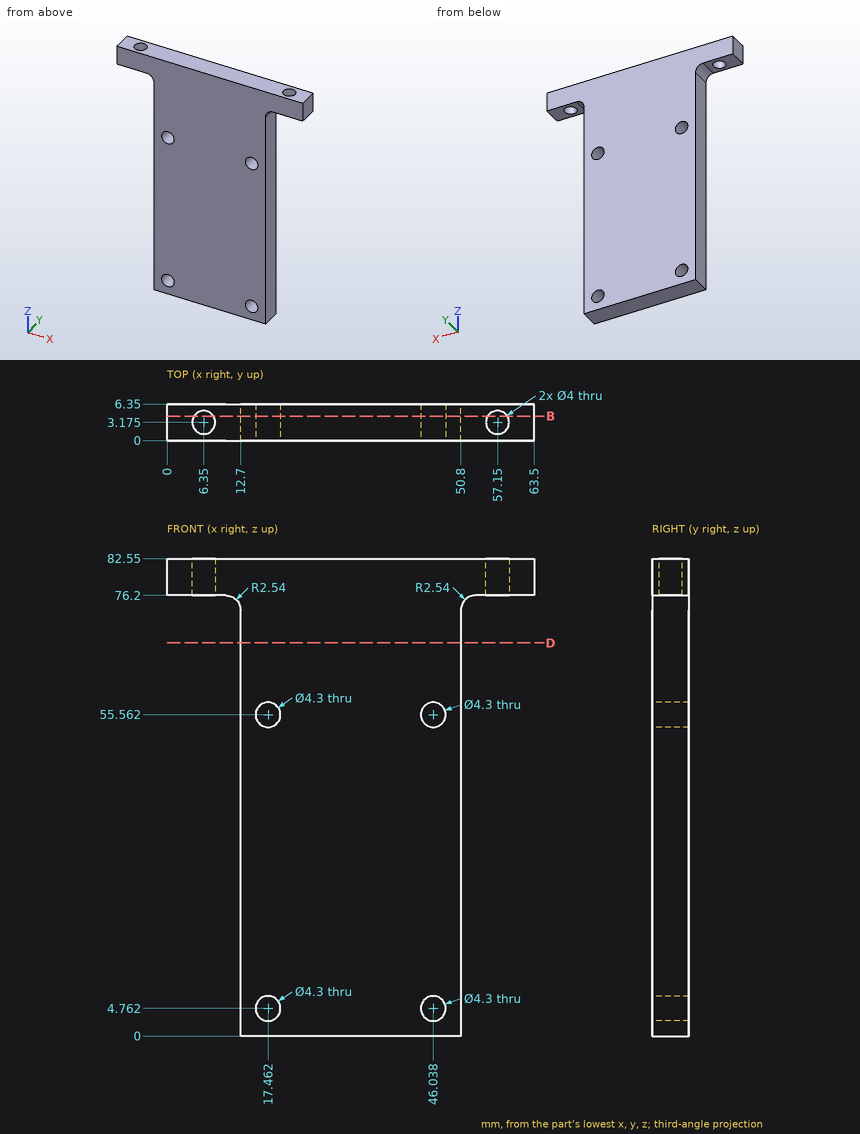
Geometry: see drawing. Coordinates: mm, zero at the bounding-box minimum. Round coordinates to 2 decimals unless told otherwise and drop trailing zeros. Write each loop counter-clockwise with the first axis right and the second up, starting at its lowest first coordinate (ties: lowest second). Pieces come first, ordered by that corner, then holes. Notation, with made-up numbers: (-1, 22.25) - (52, 22.25) arc R18 cw to (52, 48.25) - close; hole circle Ø9 at (29.25, 9). An arc over 180 degrees is marked (long way). Use CSV: the item, a comma, the result in double quotes. Start each with the question number.
(1) First-contact query: pin 1 Ø3.5 at (x, z) = (17.46, 55.56) entering from -Y; pin 2 Ø3 at (x, y) = (3.5, 2) entering from -Z; pin 3 Ø1.9 at (y, z) = (2, 48.5) entering from +X. Flat tips, straight axial feed; report the tip coordinate or a pass-through.
(2) Material intervals for probe 1 along Z at (x, y) = (46, 5.5); probe 2 along X at (y, z) = (2, 57) (1 decimal); probe 3 along X at (y, z) = (3.75, 16), sorted ascending. Write a range as [from, to].
(3) Cut plane B-B, the plane y = 4.25. Return loops of the section in (x, z), and give its area (3 significant figures).
(4) Cut plane D-D, the plane z = 68. Return loops of the section in (x, y), and give its area (3 significant figures).
Geometry says:
1,pin 1,"through"
1,pin 2,"z = 76.2"
1,pin 3,"x = 50.8"
2,probe 1,"[0, 2.61], [6.91, 53.41], [57.71, 82.55]"
2,probe 2,"[12.7, 15.9], [19.1, 44.4], [47.6, 50.8]"
2,probe 3,"[12.7, 50.8]"
3,outline,"(0, 76.2) - (4.66, 76.2) - (4.66, 82.55) - (0, 82.55) - close; (8.04, 76.2) - (10.16, 76.2) arc R2.54 cw to (12.7, 73.66) - (12.7, 0) - (50.8, 0) - (50.8, 73.66) arc R2.54 cw to (53.34, 76.2) - (55.46, 76.2) - (55.46, 82.55) - (8.04, 82.55) - close; (58.84, 76.2) - (63.5, 76.2) - (63.5, 82.55) - (58.84, 82.55) - close; hole circle Ø4.3 at (17.46, 4.76); hole circle Ø4.3 at (17.46, 55.56); hole circle Ø4.3 at (46.04, 4.76); hole circle Ø4.3 at (46.04, 55.56)"
3,area,"3,210 mm²"
4,outline,"(12.7, 0) - (50.8, 0) - (50.8, 6.35) - (12.7, 6.35) - close"
4,area,"242 mm²"
